Print and shaded views of the part. All mm, measured from the part's lowest x, y and z. Coordinates: 2 decimals unless noted, no trailing zeros. Loops run counter-clockwise (first coordinate to the right, second up) from the corner with the lowest first, then second, coordinate; pieces in that order, holes last. Notation, with made-up numbers: M -14,-4.5 L 35,-4.5 A19 cw 35,14.5 Z; hole C 17,36 d8. An arc over 180 degrees is marked long. Use a Markdown table: item, result. Add a question column.
1) Band-saw the part on C-C (z = 6). List the corners of the cut face in (x, y), plus the area to 3 significant figures.
2) Band-saw the part on D-D (x = 950). List the corners of the cut face in (y, z), plus the area to 3 significant figures.
3) Band-saw the part on B-B (x = 640). List the corners of the cut face in (y, z).
4) Wall check: probe 1 along X at (y, z) = (267.5, 1.5); probe 2 along Y at (x, z) = (640, 4.75); probe 3 along X at (y, z) = (202, 2.5). Give the ranges that are in metal, low to high. Write a range as from..to.
5) Band-saw the part on A-A (y = 272.5). List the corners of the cut face in (x, z).
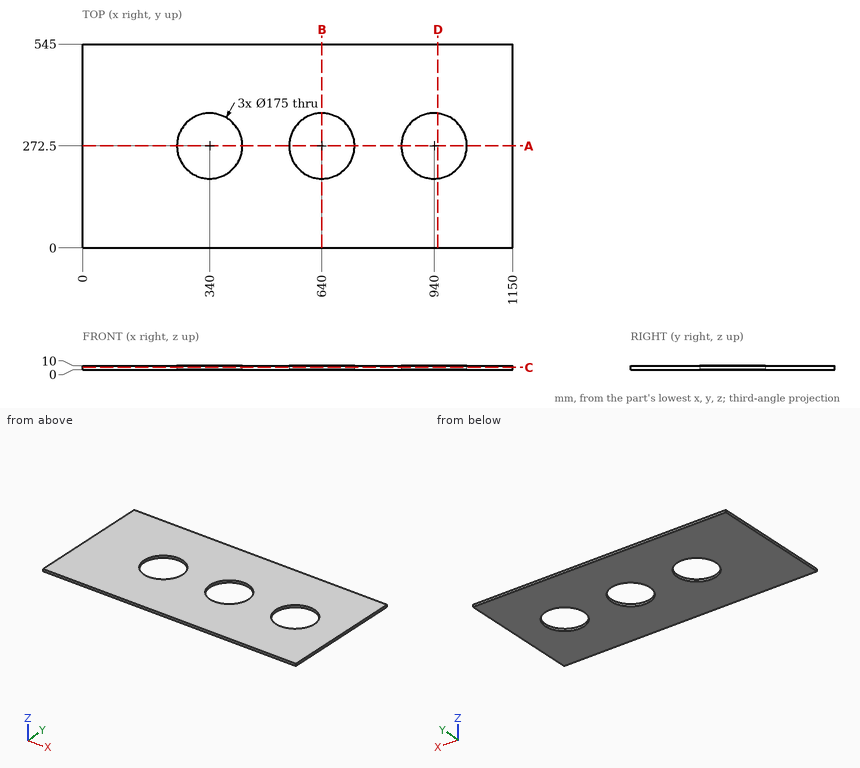
Entries:
| question | item | result |
|---|---|---|
| 1 | outline | M 0,0 L 1150,0 L 1150,545 L 0,545 Z; hole C 340,272.5 d175; hole C 640,272.5 d175; hole C 940,272.5 d175 |
| 1 | area | 555,000 mm2 |
| 2 | outline | M 0,0 L 185.57,0 L 185.57,10 L 0,10 Z; M 359.43,0 L 545,0 L 545,10 L 359.43,10 Z |
| 2 | area | 3,710 mm2 |
| 3 | outline | M 0,0 L 185,0 L 185,10 L 0,10 Z; M 360,0 L 545,0 L 545,10 L 360,10 Z |
| 4 | probe 1 | 0..252.64, 427.36..552.64, 727.36..852.64, 1027.36..1150 |
| 4 | probe 2 | 0..185, 360..545 |
| 4 | probe 3 | 0..288.17, 391.83..588.17, 691.83..888.17, 991.83..1150 |
| 5 | outline | M 0,0 L 252.5,0 L 252.5,10 L 0,10 Z; M 427.5,0 L 552.5,0 L 552.5,10 L 427.5,10 Z; M 727.5,0 L 852.5,0 L 852.5,10 L 727.5,10 Z; M 1027.5,0 L 1150,0 L 1150,10 L 1027.5,10 Z |
